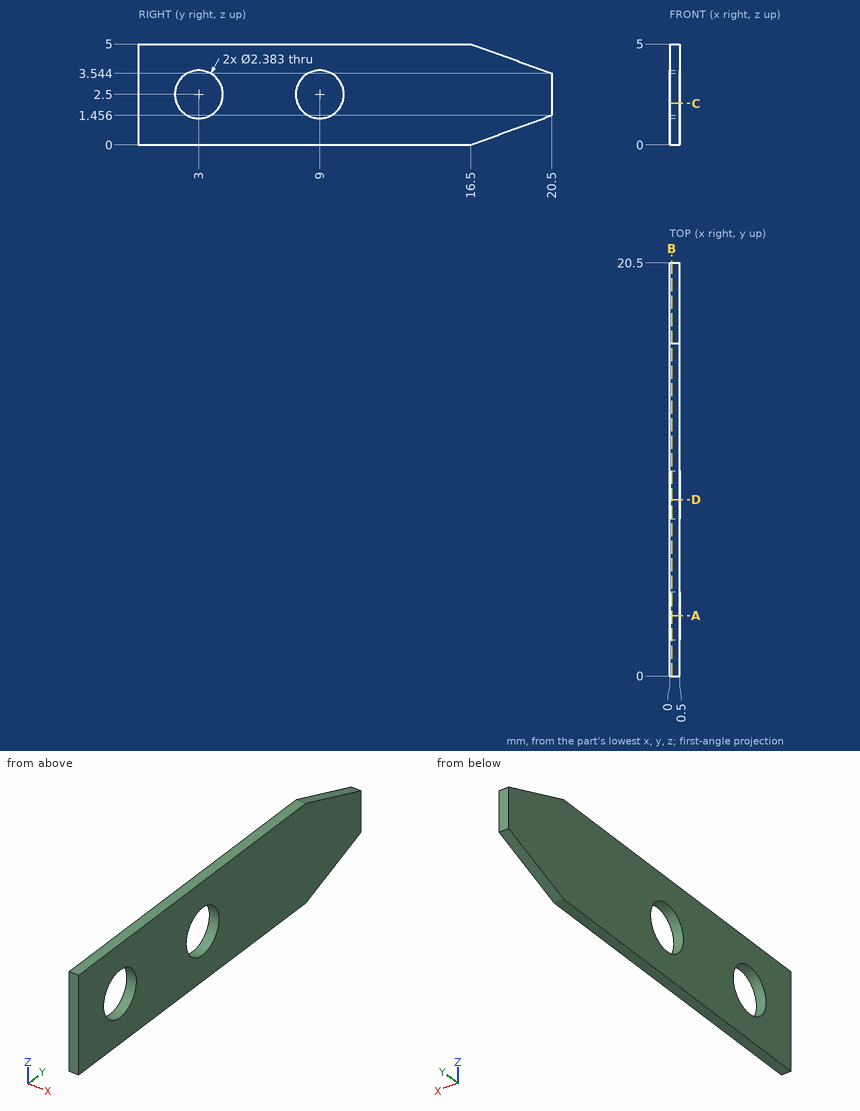
Job drawing, mm, ordinate dimensions from the low corner. One solid piece. Coordinates: 2 decimals unless noted, no trailing zeros. Write each loop counter-clockwise with the first axis right and the second up, starting at its lowest first coordinate (ties: lowest second). Pieces come first, ordered by that corner, then holes.
Item 1: Slice it at D-D (y = 8.75). Write the cut outline in (x, z) (1 decimal).
Item 2: Slice it at C-C (z = 2.05). Write the cut outline in (x, y).
Item 3: Pin check, flat tip, straight feed: pin 1 (1.4 mm diameter, centred on y = 9, z = 2.5, fed in from +X). Stop position of the tip, or through.
Item 4: Slice it at A-A (y = 3). Write the cut outline in (x, z).
Item 5: Slice it at B-B (x = 0.1). Write the cut outline in (y, z) (1 decimal).
Item 6: Probe line 1 (Y direction, x = 0.2, z = 2.5); line 2 (Y direction, x = 0.1, z = 3.1); line 3 (Z direction, x = 0.35, y = 3.75) (1 decimal). List the from-to ranges inside material, lowest first.
Results found:
1. outline: (0, 0) - (0.5, 0) - (0.5, 1.3) - (0, 1.3) - close; (0, 3.7) - (0.5, 3.7) - (0.5, 5) - (0, 5) - close
2. outline: (0, 0) - (0.5, 0) - (0.5, 1.9) - (0, 1.9) - close; (0, 4.1) - (0.5, 4.1) - (0.5, 7.9) - (0, 7.9) - close; (0, 10.1) - (0.5, 10.1) - (0.5, 20.5) - (0, 20.5) - close
3. pin 1: passes through
4. outline: (0, 0) - (0.5, 0) - (0.5, 1.31) - (0, 1.31) - close; (0, 3.69) - (0.5, 3.69) - (0.5, 5) - (0, 5) - close
5. outline: (0, 0) - (16.5, 0) - (20.5, 1.5) - (20.5, 3.5) - (16.5, 5) - (0, 5) - close; hole circle Ø2.4 at (3, 2.5); hole circle Ø2.4 at (9, 2.5)
6. line 1: y = 0 to 1.81, 4.19 to 7.81, 10.19 to 20.5
6. line 2: y = 0 to 1.97, 4.03 to 7.97, 10.03 to 20.5
6. line 3: z = 0 to 1.6, 3.4 to 5
